```python
from build123d import *

# Parameters (mm, degrees)
EXTRUDE_436_DEPTH = 5
FILLET_R_R        = 3


with BuildPart() as part:
    # ｽｹｯﾁ1 → Extrude 436 (new, symmetric)
    with BuildSketch(Plane.XY):
        Polygon((-22, -22), (100, -22), (100, -8), (22, 22), (-22, 22), align=None)
    extrude(amount=EXTRUDE_436_DEPTH, both=True)

    # 角R
    fillet_r_edges = [part.edges().sort_by_distance(p)[0] for p in [
        (-22, 22, 0),
        (22, 22, 0),
        (100, -8, 0),
        (100, -22, 0),
        (-22, -22, 0),
    ]]
    fillet(fillet_r_edges, radius=FILLET_R_R)


solid = part.part
```
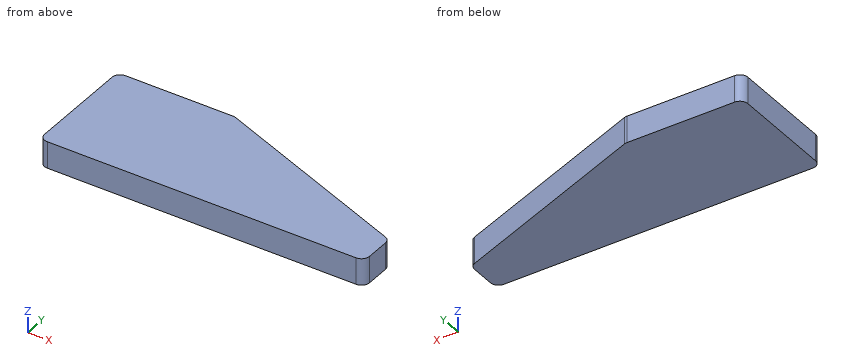
Design review of the part built by this model. Coordinates are the model's own, in mm. Round coordinates to 2 decimals unless told otherwise and drop trailing zeros. Write each loop counter-clockwise with the first axis right and the second up, starting at its lowest first coordinate (ties: lowest second). Pieces come first, ordered by that corner, then holes. Notation, with made-up numbers: (53, 32) -> (83, 32) arc R21 ccw to (83, 56) -> close; hole circle Ø7 at (54, -26.5). An arc over 180 degrees is marked (long way). Answer in a Markdown table with one row per item.
Q1. Take a section at C-C, the plane x = 58. State the section outline as (y, z) points.
The answers:
| item | result |
|---|---|
| outline | (-22, -5) -> (8.15, -5) -> (8.15, 5) -> (-22, 5) -> close |
Q2. Take a section at A-A, the plane z = 0.25. State the section outline as (x, y) points, then the cut area to 3 significant figures.
The answers:
| item | result |
|---|---|
| outline | (-22, -19) arc R3 ccw to (-19, -22) -> (97, -22) arc R3 ccw to (100, -19) -> (100, -10.06) arc R3 ccw to (98.08, -7.26) -> (22.52, 21.8) arc R3 ccw to (21.44, 22) -> (-19, 22) arc R3 ccw to (-22, 19) -> close |
| area | 4,190 mm² |
Q3. To check wall thickness, follow L1, parallel to Y at x = 23.5, z = -0.25; L2, parallel to Y at x = 33, z = -2.5. State the ranges of each line that lie inside material, in increasing order. Write a range as [from, to].
The answers:
| item | result |
|---|---|
| L1 | [-22, 21.42] |
| L2 | [-22, 17.77] |
Q4. Take a section at B-B, the plane y = 15.5. State the section outline as (x, z) points.
The answers:
| item | result |
|---|---|
| outline | (-22, -5) -> (38.9, -5) -> (38.9, 5) -> (-22, 5) -> close |
